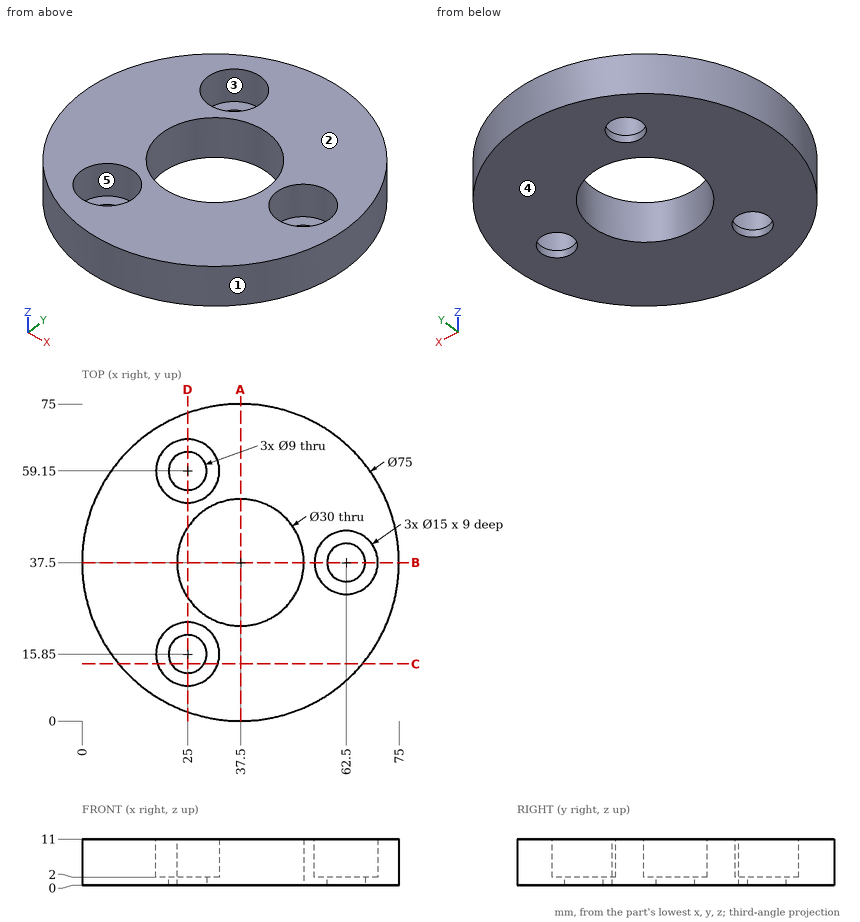
Part print with two shaded views. Sizes in mm from the minimum x, y, z corner. A direction names the side the tool comes from. Coordinates: 2 decimals unless noted, no trailing zeros. Loops run counter-clockwise (first coordinate to the right, second up) from the corner with the lowest first, then second, coordinate; pieces in that order, holes last. Notation, with made-up numbers: (87.5, 27) - (131.5, 27) arc R8 ccw to (131.5, 38) - close; hole circle Ø9 at (-5.75, 18). An arc over 180 degrees is marked (long way). Write each question's results on one line, items separated by ' | '. Start each with the question number.
Q1. Drop flat-ended pins along their axis: pin 1 Ø13.5 at (x, y) = (62.5, 37.5) entering from +Z; pin 2 Ø1 at (x, z) = (51.5, 4.5) entering from -Y; pin 3 Ø5 at (y, z) = (17, 2.5) entering from +X. Give the stop position or say it passes through.
Q2. Slice it at B-B on y = 37.5. Give the cut face in (x, z).
Q3. Slice it at C-C on y = 13.5. Give the cut face in (x, z).
Q4. Two-plate mould, pull along Y, no slides. Class the marked faces 1, 2 and 3: +Y half, -Y half, draft (parallel to the pull), parting line (faces both ways), or undercut.
Q5. Slice it at D-D on x = 25. Give the cut face in (y, z), and give its area (3 significant figures).
Q6. Slice it at A-A on x = 37.5. Give the cut face in (y, z).
Q7. Probe line 1 along Y through (x, z) = (25, 5.75); line 2 along X through (y, z) = (40.5, 5); line 3 along Y through (x, z) = (29, 7.25). List the from-to ranges inside material, lowest first.
Q8. Which spindle directions (+Z, -Z, +X, -X, +Y, -Y) get a long thin tool onto all of the face, cutting with end or side? Do the marked faces 4 and 5. Say none if no direction does.
Answer:
1) pin 1: stops at z = 2 | pin 2: stops at y = 2.51 | pin 3: stops at x = 70.4
2) outline: (0, 0) - (22.5, 0) - (22.5, 11) - (0, 11) - close; (52.5, 0) - (58, 0) - (58, 2) - (55, 2) - (55, 11) - (52.5, 11) - close; (67, 0) - (75, 0) - (75, 11) - (70, 11) - (70, 2) - (67, 2) - close
3) outline: (8.69, 0) - (21.16, 0) - (21.16, 2) - (17.88, 2) - (17.88, 11) - (8.69, 11) - close; (28.84, 0) - (66.31, 0) - (66.31, 11) - (32.12, 11) - (32.12, 2) - (28.84, 2) - close
4) face 1: parting line | face 2: draft | face 3: undercut
5) outline: (2.14, 0) - (11.35, 0) - (11.35, 2) - (8.35, 2) - (8.35, 11) - (2.14, 11) - close; (20.35, 0) - (29.21, 0) - (29.21, 11) - (23.35, 11) - (23.35, 2) - (20.35, 2) - close; (45.79, 0) - (54.65, 0) - (54.65, 2) - (51.65, 2) - (51.65, 11) - (45.79, 11) - close; (63.65, 0) - (72.86, 0) - (72.86, 11) - (66.65, 11) - (66.65, 2) - (63.65, 2) - close | area: 289 mm2
6) outline: (0, 0) - (22.5, 0) - (22.5, 11) - (0, 11) - close; (52.5, 0) - (75, 0) - (75, 11) - (52.5, 11) - close
7) line 1: y = 2.14 to 8.35, 23.35 to 29.21, 45.79 to 51.65, 66.65 to 72.86 | line 2: x = 0.12 to 22.8, 52.2 to 55.63, 69.37 to 74.88 | line 3: y = 0.98 to 9.51, 22.19 to 25.14, 49.86 to 52.81, 65.49 to 74.02
8) face 4: -Z, +X, -X, +Y, -Y | face 5: +Z
